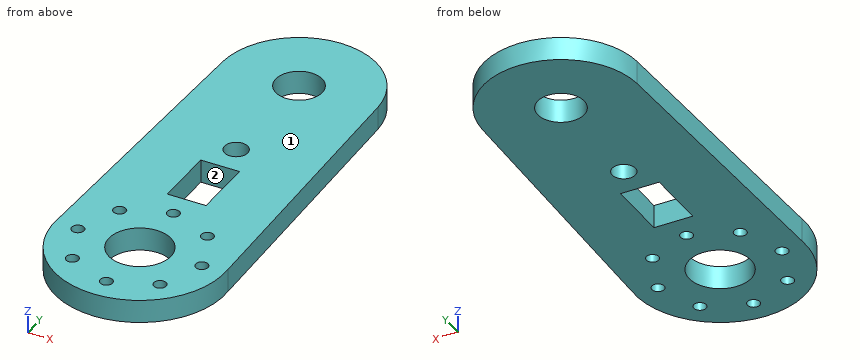
from build123d import *

# Parameters (mm, degrees)
IZIM1_R                     = 0.8
IZIM1_R_2                   = 3
IZIM1_R_3                   = 4
IZIM1_R_4                   = 1.5
IZIM1_W                     = 5
IZIM1_H                     = 8
Y_KSEKLIK_EKSTR_ZYON1_DEPTH = 3


with BuildPart() as part:
    # Çizim1 → Yükseklik-Ekstrüzyon1 (new body)
    with BuildSketch(Plane.XY.offset(3)):
        with BuildLine():
            Line((10.975849913, 0.728504421), (9.994509837, 38.331320273))
            ThreePointArc((9.994509837, 38.331320273), (0, 48), (-9.994509837, 38.331320273))
            Line((-9.994509837, 38.331320273), (-10.975849913, 0.728504421))
            ThreePointArc((-10.975849913, 0.728504421), (0, -11), (10.975849913, 0.728504421))
        make_face()
        with Locations((0, 8)):
            Circle(IZIM1_R, mode=Mode.SUBTRACT)
        with Locations((5.656854249, 5.656854249)):
            Circle(IZIM1_R, mode=Mode.SUBTRACT)
        with Locations((8, 0)):
            Circle(IZIM1_R, mode=Mode.SUBTRACT)
        with Locations((5.656854249, -5.656854249)):
            Circle(IZIM1_R, mode=Mode.SUBTRACT)
        with Locations((0, -8)):
            Circle(IZIM1_R, mode=Mode.SUBTRACT)
        with Locations((-5.656854249, -5.656854249)):
            Circle(IZIM1_R, mode=Mode.SUBTRACT)
        with Locations((-8, 0)):
            Circle(IZIM1_R, mode=Mode.SUBTRACT)
        with Locations((0, 38)):
            Circle(IZIM1_R_2, mode=Mode.SUBTRACT)
        Circle(IZIM1_R_3, mode=Mode.SUBTRACT)
        with Locations((0, 23)):
            Circle(IZIM1_R_4, mode=Mode.SUBTRACT)
        with Locations((-5.656854249, 5.656854249)):
            Circle(IZIM1_R, mode=Mode.SUBTRACT)
        with Locations((0, 15.169050412)):
            Rectangle(IZIM1_W, IZIM1_H, mode=Mode.SUBTRACT)
    extrude(amount=-Y_KSEKLIK_EKSTR_ZYON1_DEPTH)


solid = part.part
The listing builds one solid part. Answer for the finished solid, in the listing's coordinates (mm). Face numbers are marked on the shaded views. A direction names the side the tool comes from. Coordinates: 2 decimals unless noted, no trailing zeros. Loops run counter-clockwise (first coordinate to the right, second up) from the corner with the lowest first, then second, coordinate; pieces in that order, holes last. Notation, with made-up numbers: (81.25, 42.5) -> (139.25, 42.5) arc R26 cw to (139.25, 79.5) -> close; hole circle Ø2 at (84.25, 49.25). An arc over 180 degrees is marked (long way). Write item = value, one per line. Start each with the question number.
1) A cutting plane is placed at D-D (z = 0.7). Count the separate pieces of the cut face and the enclosed holes in it, then the cut area to 3 significant figures.
2) Given pin 1 Ø1 at (y, z) = (5.5, 1) entering from -X; pin 2 Ø1 at (y, z) = (16, 1.5) entering from +X, each flat-ended and moving along its own axis, determine where each tip first touches the part or whether it passes through.
3) A cutting plane is placed at A-A (y = 0). Give the vertices of the cut face in (x, z).
4) A cutting plane is placed at B-B (x = 7.75). Give the vertices of the cut face in (y, z).
5) A tool of negligible diameter and unlimited length cuts with its end or side. For the marked faces 1 and 2, from which of +Z, -Z, +X, -X, +Y, -Y can it reach the whole face along a straight path? Write none if from no direction.
6) Straight lines are drawn through the part: line 1 (Y direction, x = -1.75, z = 0.4); line 2 (X direction, y = -5.5, z = 0.2); line 3 (Y direction, x = -3.25, z = 1.25). For each, find the intervals that lie inside material, in ascending order. Write a range as from..to.
7) A cutting plane is placed at C-C (y = 8). Give the vertices of the cut face in (x, z), then the cut area to 3 significant figures.
Responses:
q1.separate_pieces = 1
q1.enclosed_holes = 12
q1.area = 1,000 mm²
q2.pin_1 = -10.86
q2.pin_2 = 10.59
q3.outline = (-11, 0) -> (-8.8, 0) -> (-8.8, 3) -> (-11, 3) -> close; (-7.2, 0) -> (-4, 0) -> (-4, 3) -> (-7.2, 3) -> close; (4, 0) -> (7.2, 0) -> (7.2, 3) -> (4, 3) -> close; (8.8, 0) -> (11, 0) -> (11, 3) -> (8.8, 3) -> close
q4.outline = (-7.81, 0) -> (-0.76, 0) -> (-0.76, 3) -> (-7.81, 3) -> close; (0.76, 0) -> (44.32, 0) -> (44.32, 3) -> (0.76, 3) -> close
q5.face_1 = +Z, +X, -X, +Y, -Y
q5.face_2 = +Z, -Z
q6.line_1 = -10.86..-3.6, 3.6..11.17, 19.17..35.56, 40.44..47.85
q6.line_2 = -9.53..-6.44, -4.87..4.87, 6.44..9.53
q6.line_3 = -10.51..-2.33, 2.33..47.46
q7.outline = (-10.79, 0) -> (-0.8, 0) -> (-0.8, 3) -> (-10.79, 3) -> close; (0.8, 0) -> (10.79, 0) -> (10.79, 3) -> (0.8, 3) -> close
q7.area = 59.9 mm²
